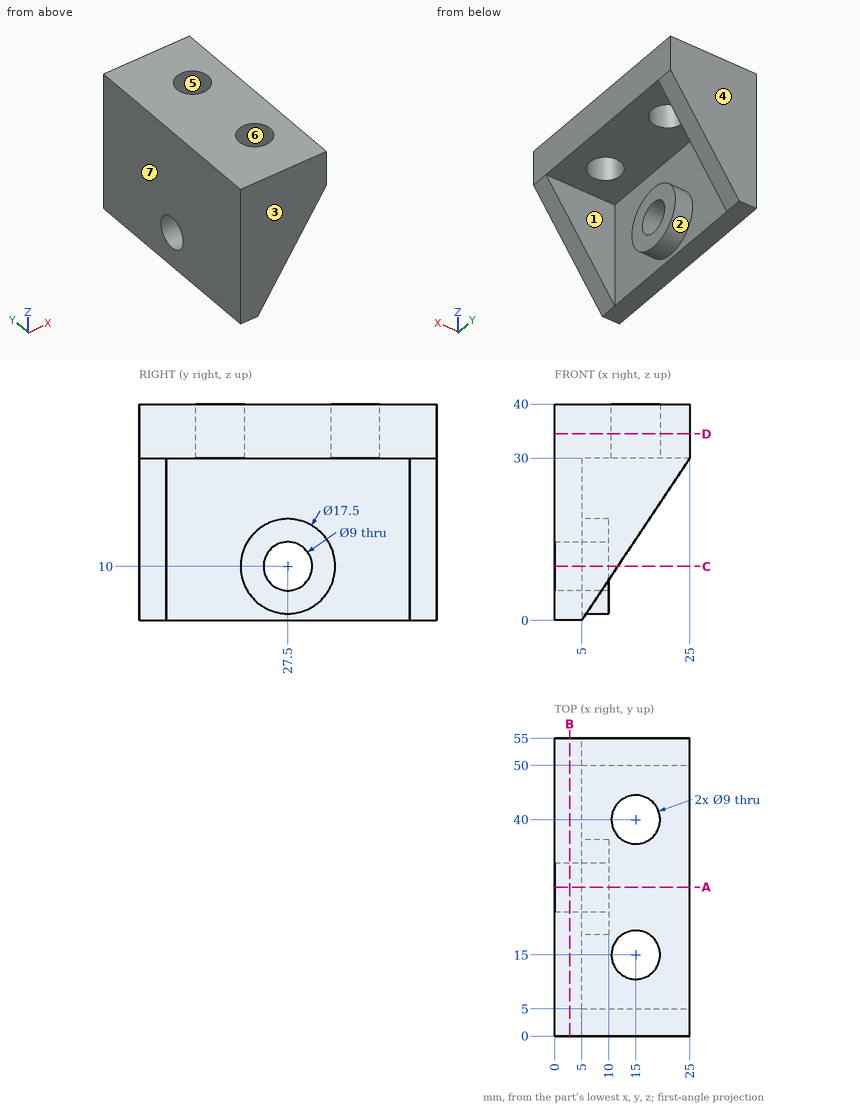
The drawing under review shows one solid part. Ordinate dimensions are in mm from its lowest x, y, z. A direction names the side the tool comes from. Give positions to 0.01 mm unless a question says otherwise; leave off trailing zeros. Write each loop counter-clockwise with the first axis right and the second up, starting at its lowest first coordinate (ties: lowest second). Pieces come first, ordered by that corner, then holes. Notation, with made-up numbers: (14.5, 33) - (41.5, 33) arc R29 ccw to (41.5, 54) - close; hole circle Ø2 at (43, 35.25). An arc over 180 degrees is marked (long way). Answer in a Markdown table with one row per item. Add a question column.
1. Tool access review of the marked faces 1, 2 and 3: name each direction out of +Z, -Z, +X, -X, +Y, -Y from which nothing blocks a thin tool from reaching the whole face with its end or side.
2. Insertion check: P1, Ø8, axis at x = 15, y = 40, coming from the +Z side; P2, Ø1, axis at y = 12.5, z = 8.5, coming from the +X side; P3, Ø10, axis at x = 20, y = 26.5, coming from the -Z side; P4, Ø1, axis at x = 6, y = 35, coming from the -Z side. Each pin has a flat end and moves straight along its axis. Give the tip position at first contact, or say it passes through.
3. Wall thickness on line 1 along Y through (x, z) = (15, 35.25); line 2 along Y through (x, z) = (7.5, 10); line 3 along Y through (x, z) = (12.75, 23.5): over which ranges is each line inside the solid? List them lowest first. Write a range as [from, to].
4. We need section D-D on z = 34.5. Write out the cut boundary in (x, y).
5. We need section B-B on x = 2.75. Write out the cut boundary in (y, z), then the cut area to 3 significant figures.
6. Draft analysis for pull direction X (two halves, no side actions). For the marked faces 4, 5, 6 and 7, state which applies: +X half, -X half, draft (parallel to the pull), parting line (faces both ways), or undercut.
7. We need section C-C on z = 10. Write out the cut boundary in (x, y), then the cut area to 3 significant figures.
8. We need section A-A on y = 27.5. Write out the cut boundary in (x, z), then the cut area to 4 significant figures.
Ans:
| question | item | result |
|---|---|---|
| 1 | face 1 | -Z, +X |
| 1 | face 2 | +X |
| 1 | face 3 | +Z, -Z, +X, -X, -Y |
| 2 | P1 | passes through |
| 2 | P2 | stops at x = 5 |
| 2 | P3 | stops at z = 30 |
| 2 | P4 | stops at z = 4.75 |
| 3 | line 1 | y = [0, 10.5], [19.5, 35.5], [44.5, 55] |
| 3 | line 2 | y = [0, 5], [18.75, 23], [32, 36.25], [50, 55] |
| 3 | line 3 | y = [0, 5], [50, 55] |
| 4 | outline | (0, 0) - (25, 0) - (25, 55) - (0, 55) - close; hole circle Ø9 at (15, 15); hole circle Ø9 at (15, 40) |
| 5 | outline | (0, 0) - (55, 0) - (55, 40) - (0, 40) - close; hole circle Ø9 at (27.5, 10) |
| 5 | area | 2,140 mm^2 |
| 6 | face 4 | draft |
| 6 | face 5 | undercut |
| 6 | face 6 | undercut |
| 6 | face 7 | -X half |
| 7 | outline | (0, 0) - (11.67, 0) - (11.67, 5) - (5, 5) - (5, 18.75) - (10, 18.75) - (10, 23) - (0, 23) - close; (0, 32) - (10, 32) - (10, 36.25) - (5, 36.25) - (5, 50) - (11.67, 50) - (11.67, 55) - (0, 55) - close |
| 7 | area | 339 mm^2 |
| 8 | outline | (0, 0) - (5, 0) - (5, 1.25) - (10, 1.25) - (10, 5.5) - (0, 5.5) - close; (0, 14.5) - (10, 14.5) - (10, 18.75) - (5, 18.75) - (5, 30) - (25, 30) - (25, 40) - (0, 40) - close |
| 8 | area | 397.5 mm^2 |
